Design review of the part built by this model. Coordinates are the model's own, in mm. A direction names the side the tool comes from. Give positions to 0.01 mm unless a question says otherwise; leave off trailing zeros. Order: outer loops, then holes, each group sorted by start corner. A loop starts at its lowest first (then second) coordinate and runs counter-clockwise, first axis right, second up. Notation, with made-up numbers: (-24.5, -27) -> (-4.5, -27) arc R18 cw to (-4.5, 0) -> close; hole circle Ø4 at (40.25, 58). An arc over 180 degrees is marked (long way). Use a Markdown table: item, result. Add a question column.
```python
from build123d import *

# Parameters (mm, degrees)
SKETCH1_W                    = 127
SKETCH1_H                    = 38.1
BASE_FLANGE1_DEPTH           = 3.175
EDGE_FLANGE1_STRIP_W         = 14.1732
EDGE_FLANGE1_STRIP_H         = 3.175
EDGE_FLANGE1_STRIP_CUT_DEPTH = 127
EDGE_FLANGE1_DEPTH           = 127
SKETCH9_R                    = 3.175
SKETCH9_R_2                  = 47.625
CUT_EXTRUDE1_DEPTH           = 169.868266273
EDGE_FLANGE2_START           = -63.5
EDGE_FLANGE2_DEPTH           = 127
EDGE_FLANGE2_2_DEPTH         = 127
TAB1_DEPTH                   = 3.175
SKETCH16_R                   = 6.35
CUT_EXTRUDE2_DEPTH           = 235.714429908
BREAK_CORNER1_START          = -171.342480702
BREAK_CORNER1_OUTLINE_W      = 10
BREAK_CORNER1_OUTLINE_H      = 6
BREAK_CORNER1_DEPTH          = 5.219227672
BREAK_CORNER1_START_2        = 166.12325303
BREAK_CORNER1_2_OUTLINE_W    = 10
BREAK_CORNER1_2_OUTLINE_H    = 6
BREAK_CORNER1_2_DEPTH        = 5.219227672
BREAK_CORNER1_START_3        = 53.881536726
BREAK_CORNER1_3_OUTLINE_W    = 12
BREAK_CORNER1_3_OUTLINE_H    = 6
BREAK_CORNER1_3_DEPTH        = 4.490128061
BREAK_CORNER1_START_4        = -58.371664787
BREAK_CORNER1_4_OUTLINE_W    = 12
BREAK_CORNER1_4_OUTLINE_H    = 6
BREAK_CORNER1_4_DEPTH        = 4.490128061
SKETCH17_R                   = 4.7625
CUT_EXTRUDE3_DEPTH           = 239.261598489


# Read off the part's stored shape, not the designer's step: Edge-Flange2, Break-Corner1
# Sheet-metal steps are written as plain solids
with BuildPart() as part:
    # Sketch1 → Base-Flange1 (new body)
    with BuildSketch(Plane.XY):
        Rectangle(SKETCH1_W, SKETCH1_H)
    extrude(amount=-BASE_FLANGE1_DEPTH)

    # Edge-Flange1 strip (across the edge) → Edge-Flange1 strip cut (cut)
    with BuildSketch(Plane(origin=(-63.5, -19.05, 0), x_dir=(0, 1, 0), z_dir=(1, 0, 0))):
        with Locations((-3.175, -1.5875)):
            Rectangle(EDGE_FLANGE1_STRIP_W, EDGE_FLANGE1_STRIP_H)
    extrude(amount=EDGE_FLANGE1_STRIP_CUT_DEPTH, mode=Mode.SUBTRACT)

    # Edge-Flange1 section (across the edge) → Edge-Flange1 (add)
    with BuildSketch(Plane(origin=(-63.5, -19.05, 0), x_dir=(0, 1, 0), z_dir=(1, 0, 0))):
        with BuildLine():
            Line((0, 0.7366), (0, 152.527))
            Line((0, 152.527), (3.175, 152.527))
            Line((3.175, 152.527), (3.175, 0.7366))
            ThreePointArc((3.175, 0.7366), (3.390745145, 0.215745145), (3.9116, 0))
            Line((3.9116, 0), (3.9116, -3.175))
            ThreePointArc((3.9116, -3.175), (1.145681115, -2.029318885), (0, 0.7366))
        make_face()
    extrude(amount=EDGE_FLANGE1_DEPTH)

    # Sketch9 → Cut-Extrude1 (cut, through all)
    with BuildSketch(Plane(origin=(0, -15.875, 0), x_dir=(1, 0, 0), z_dir=(0, 1, 0))):
        with Locations(Location((0, -6.985, 0), (0, 0, 270))):
            Circle(SKETCH9_R)
        with Locations(Location((38.166088515, -22.793911485, 0), (0, 0, 270))):
            Circle(SKETCH9_R)
        with Locations(Location((53.975, -60.96, 0), (0, 0, 270))):
            Circle(SKETCH9_R)
        with Locations(Location((38.166088515, -99.126088515, 0), (0, 0, 270))):
            Circle(SKETCH9_R)
        with Locations(Location((0, -114.935, 0), (0, 0, 270))):
            Circle(SKETCH9_R)
        with Locations(Location((-38.166088515, -99.126088515, 0), (0, 0, 270))):
            Circle(SKETCH9_R)
        with Locations(Location((-53.975, -60.96, 0), (0, 0, 270))):
            Circle(SKETCH9_R)
        with Locations(Location((-38.166088515, -22.793911485, 0), (0, 0, 270))):
            Circle(SKETCH9_R)
        with Locations(Location((0, -60.96, 0), (0, 0, 270))):
            Circle(SKETCH9_R_2)
    extrude(amount=-CUT_EXTRUDE1_DEPTH, mode=Mode.SUBTRACT)

    # Edge-Flange2 outline → Edge-Flange2 (cut)
    with BuildSketch(Plane.YZ.offset(EDGE_FLANGE2_START)):
        with BuildLine():
            ThreePointArc((-19.05, 148.674785068), (-18.241680926, 151.056016274), (-16.150796577, 152.45310053))
            Line((-16.150796577, 152.45310053), (-15.875, 152.527))
            Line((-15.875, 152.527), (-19.05, 152.527))
            Line((-19.05, 152.527), (-19.05, 148.674785068))
        make_face()
    extrude(amount=EDGE_FLANGE2_DEPTH, mode=Mode.SUBTRACT)

    # Edge-Flange2 2 outline → Edge-Flange2 2 (add)
    with BuildSketch(Plane.YZ.offset(EDGE_FLANGE2_START)):
        with BuildLine():
            Line((109.756208936, 186.189780978), (-15.875, 152.527))
            Line((-15.875, 152.527), (-15.875, 148.674785068))
            ThreePointArc((-15.875, 148.674785068), (-15.72278407, 149.123198736), (-15.329046109, 149.386286031))
            Line((-15.329046109, 149.386286031), (110.577959404, 183.12296648))
            Line((110.577959404, 183.12296648), (109.756208936, 186.189780978))
        make_face()
    extrude(amount=EDGE_FLANGE2_2_DEPTH)

    # Sketch13 → Tab1 (add)
    with BuildSketch(Plane(origin=(0, -39.195173357, 146.278378382), x_dir=(1, 0, 0), z_dir=(0, -0.258819045102528, 0.9659258262890663))):
        Polygon((-63.5, 154.205818127), (-101.6, 154.205818127), (-63.5, 52.605818127), align=None)
        Polygon((101.6, 154.205818127), (63.5, 52.605818127), (63.5, 154.205818127), align=None)
    extrude(amount=-TAB1_DEPTH)

    # Sketch16 → Cut-Extrude2 (cut, through all)
    with BuildSketch(Plane(origin=(0, -39.195173357, 146.278378382), x_dir=(1, 0, 0), z_dir=(0, -0.258819045102528, 0.9659258262890663))):
        with Locations(Location((69.85, 134.705637142, 0), (0, 0, 270))):
            Circle(SKETCH16_R)
        with Locations(Location((-69.85, 134.705637142, 0), (0, 0, 270))):
            Circle(SKETCH16_R)
    extrude(amount=-CUT_EXTRUDE2_DEPTH, mode=Mode.SUBTRACT)

    # Break-Corner1 outline → Break-Corner1 (cut)
    with BuildSketch(Plane(origin=(0, 0, 0), x_dir=(0.5695948377626004, 0.7939191812855688, 0.212730003481053), z_dir=(0.8219256175556257, -0.5501863643158269, -0.14742199200504597)).offset(BREAK_CORNER1_START)):
        with Locations((69, 150)):
            Rectangle(BREAK_CORNER1_OUTLINE_W, BREAK_CORNER1_OUTLINE_H)
    extrude(amount=BREAK_CORNER1_DEPTH, mode=Mode.SUBTRACT)

    # Break-Corner1 2 outline → Break-Corner1 2 (cut)
    with BuildSketch(Plane(origin=(0, 0, 0), x_dir=(0.5695948377626027, -0.7939191812855675, -0.21273000348105187), z_dir=(0.8219256175556241, 0.5501863643158292, 0.14742199200504602)).offset(BREAK_CORNER1_START_2)):
        with Locations((-69, -150)):
            Rectangle(BREAK_CORNER1_2_OUTLINE_W, BREAK_CORNER1_2_OUTLINE_H)
    extrude(amount=BREAK_CORNER1_2_DEPTH, mode=Mode.SUBTRACT)

    # Break-Corner1 3 outline → Break-Corner1 3 (cut)
    with BuildSketch(Plane(origin=(0, 0, 0), x_dir=(0.707106781186548, -0.707106781186547, 0), z_dir=(0.707106781186547, 0.707106781186548, 0)).offset(BREAK_CORNER1_START_3)):
        with Locations((31, 2)):
            Rectangle(BREAK_CORNER1_3_OUTLINE_W, BREAK_CORNER1_3_OUTLINE_H)
    extrude(amount=BREAK_CORNER1_3_DEPTH, mode=Mode.SUBTRACT)

    # Break-Corner1 4 outline → Break-Corner1 4 (cut)
    with BuildSketch(Plane(origin=(0, 0, 0), x_dir=(0.7071067811865474, 0.7071067811865477, 0), z_dir=(0.7071067811865476, -0.7071067811865476, 0)).offset(BREAK_CORNER1_START_4)):
        with Locations((-31, -2)):
            Rectangle(BREAK_CORNER1_4_OUTLINE_W, BREAK_CORNER1_4_OUTLINE_H)
    extrude(amount=BREAK_CORNER1_4_DEPTH, mode=Mode.SUBTRACT)

    # Sketch17 → Cut-Extrude3 (cut, through all)
    with BuildSketch(Plane.XY):
        with Locations((44.45, 0)):
            Circle(SKETCH17_R)
        with Locations((-44.45, 0)):
            Circle(SKETCH17_R)
    extrude(amount=-CUT_EXTRUDE3_DEPTH, mode=Mode.SUBTRACT)


solid = part.part
```
1) Machinability: for faces 4 (the cylindrical face through (0.954, -17.44, 117.963)), 5 (the flat face through (60.3, 15.9, -1.6)), 6 (the flat face through (-1, 2, 0)), which of the approach directions +Z, -Z, +X, -X, +Y, -Y give a long, thin tool a straight path to every point of the face, cutting with its end or side? Answer none if there is none.
2) Add section C-C (y = 0). Give the boundary of the cut face in (x, z) (1 decimal), then the cut area to 3 significant figures.
3) Add section B-B (z = 41). Give the boundary of the cut face in (x, y) (3 decimals).
4) The part is to be moulded in two halves that separate along X. For faces 1 (the cylindrical face through (39.692, 0.209, -1.565)), 2 (the flat face through (-15, -19.05, 107)), 3 (the flat face through (97.28, 107.34, 183.88)), say which applies: +X half, -X half, draft (parallel to the pull), parting line (faces both ways), or undercut.
5) Insertion check: pin 1 (8.5 mm diameter, centred on x = 38.17, z = 22.79, fed in from +Y) (3 decimals); pin 2 (3 mm diameter, centred on x = -65.5, y = 80.5, fed in from -Z); pin 3 (8.5 mm diameter, centred on x = -44.45, y = 0, fed in from +Z). Each pin has a flat end and moves straight along its axis. Give the tip position at first contact, or say it passes through.
6) Add section A-A (x = 0). Give the boundary of the cut face in (y, z) (3 decimals), then the cut area to 3 significant figures.
7) Add section D-D (x = 44). Give the boundary of the cut face in (y, z) (3 decimals).
8) For L1, parallel to X at y = -17, z = 60; L2, parallel to Z at x = -23.5, y = -12 (3 decimals); L3, parallel to Y at x = -33, z = 124.5 (3 decimals), list the stretches that pass through material, from the lowest coordinate up. Write a range as [from, to].
Worked answers:
| question | item | result |
|---|---|---|
| 1 | face 4 | +Y, -Y |
| 1 | face 5 | -Z, +X, +Y |
| 1 | face 6 | +X, -X, +Y |
| 2 | outline | (-63.5, -3.2) -> (-49.2, -3.2) -> (-49.2, 0) -> (-63.5, 0) -> close; (-63.5, 153.5) -> (63.5, 153.5) -> (63.5, 156.8) -> (-63.5, 156.8) -> close; (-39.7, -3.2) -> (39.7, -3.2) -> (39.7, 0) -> (-39.7, 0) -> close; (49.2, -3.2) -> (63.5, -3.2) -> (63.5, 0) -> (49.2, 0) -> close |
| 2 | area | 760 mm^2 |
| 3 | outline | (-63.5, -19.05) -> (-43.24, -19.05) -> (-43.24, -15.875) -> (-63.5, -15.875) -> close; (43.24, -19.05) -> (63.5, -19.05) -> (63.5, -15.875) -> (43.24, -15.875) -> close |
| 4 | face 1 | undercut |
| 4 | face 2 | draft |
| 4 | face 3 | +X half |
| 5 | pin 1 | y = -15.875 |
| 5 | pin 2 | z = 174.66 |
| 5 | pin 3 | z = 157.92 |
| 6 | outline | (-19.05, 0.737) arc R3.912 ccw to (-15.138, -3.175) -> (19.05, -3.175) -> (19.05, 0) -> (-15.138, 0) arc R0.737 cw to (-15.875, 0.737) -> (-15.875, 3.81) -> (-19.05, 3.81) -> close; (-19.05, 10.16) -> (-15.875, 10.16) -> (-15.875, 13.335) -> (-19.05, 13.335) -> close; (-19.05, 108.585) -> (-15.875, 108.585) -> (-15.875, 111.76) -> (-19.05, 111.76) -> close; (-19.05, 118.11) -> (-15.875, 118.11) -> (-15.875, 148.675) arc R0.737 cw to (-15.329, 149.386) -> (110.578, 183.123) -> (109.756, 186.19) -> (-16.151, 152.453) arc R3.912 ccw to (-19.05, 148.675) -> close |
| 6 | area | 671 mm^2 |
| 7 | outline | (-19.05, 0.737) arc R3.912 ccw to (-15.138, -3.175) -> (-4.741, -3.175) -> (-4.741, 0) -> (-15.138, 0) arc R0.737 cw to (-15.875, 0.737) -> (-15.875, 42.735) -> (-19.05, 42.735) -> close; (-19.05, 79.185) -> (-15.875, 79.185) -> (-15.875, 148.675) arc R0.737 cw to (-15.329, 149.386) -> (110.578, 183.123) -> (109.756, 186.19) -> (-16.151, 152.453) arc R3.912 ccw to (-19.05, 148.675) -> close; (4.741, -3.175) -> (19.05, -3.175) -> (19.05, 0) -> (4.741, 0) -> close |
| 8 | L1 | [-63.5, -57], [-50.95, -47.62], [47.62, 50.95], [57, 63.5] |
| 8 | L2 | [-3.175, 0], [150.278, 153.565] |
| 8 | L3 | [-19.05, -15.875] |
